Model file for the job. Use its own axes, mm. A direction names the side the tool comes from. Round coordinates to 2 decimals unless told otherwise and drop trailing zeros. Order: outer loops, then holes, each group sorted by start corner. A loop starts at its lowest first (then second) coordinate and runs counter-clockwise, first axis right, second up. Notation, with made-up numbers: (39.25, -25) - (50.25, -25) arc R33 ccw to (50.25, 6) - close; hole circle Ø9 at (-23.5, 86.5). An arc over 180 degrees is marked (long way). Answer as CSV lines item,"result". Start each with the question number.
1. 3-axis set-ups, long thin cutter, end or side, ignore diameter. For faces 4 (the face through (0, 3, -35)), 5 (the face through (49.78, 5.01, 37.05)), 6 (the face through (-38.28, 8.96, 89.19)): which of +Z, -Z, +X, -X, +Y, -Y reach the whole face in a straight line?
2. Band-saw the part on B-B on x = -22. List the corners of the cut face in (y, z), then the cut area to 3 significant figures.
3. Pin check, flat tips, straight feed: pin 1 Ø8 at (x, z) = (85.56, -41.72) entering from +Y; pin 2 Ø1.5 at (x, z) = (-43, -86.5) entering from +Y. Stop position of each tip, or through.
4. Wall check: line 1 along X through (y, z) = (4.6, 0); line 2 along X through (y, z) = (3.85, -75); line 3 along Y through (x, z) = (36.5, 39.5). Give the ranges that are in metal, low to high. Write a range as [from, to].
5. Band-saw the part on A-A on z = 11. List the corners of the cut face in (x, y), then the cut area to 3 significant figures.
6. Pull direction Z, two halves, no side cores. Call faces 1 (the face through (50.48, 8.96, 90.94)), 2 (the face through (-36.342, 8.958, 76.795)), 3 (the face through (-43, 12, -82)): released by +Z, released by -Z, zero draft, split by the parting line, or undercut.
```python
from build123d import *

# Parameters (mm, degrees)
SKETCH_1_W               = 200
SKETCH_1_H               = 200
SKETCH_1_R               = 2
EXTRUDE_1_DEPTH          = 6
CUT_EXTRUDE_1_DEPTH      = 2
FILLET_1_R               = 2
EXTRUDE_3_DEPTH          = 6
FILLET_4_R               = 40
SKETCH_4_R               = 2.5
CUT_EXTRUDE_2_DEPTH      = 8
SKETCH_7_R               = 9
SKETCH_7_W               = 18
SKETCH_7_H               = 8
SKETCH_7_W_2             = 8
SKETCH_7_H_2             = 18
CUT_EXTRUDE_3_DEPTH      = 6
CUT_EXTRUDE_4_DEPTH      = 2
FILLET_6_R               = 1
CUT_EXTRUDE_5_DEPTH      = 142.548578234
CUT_EXTRUDE_5_DEPTH_BACK = 142.548578234
SKETCH_9_R               = 35


with BuildPart() as part:
    # Эскиз1 → Бобышка-Вытянуть1 (new body)
    with BuildSketch(Plane(origin=(0, 0, 0), x_dir=(1, 0, 0), z_dir=(0, 1, 0))):
        Rectangle(SKETCH_1_W, SKETCH_1_H)
        with Locations(Location((-39.5, 75, 0), (0, 0, 270))):
            Circle(SKETCH_1_R, mode=Mode.SUBTRACT)
        with Locations(Location((39.5, 75, 0), (0, 0, 270))):
            Circle(SKETCH_1_R, mode=Mode.SUBTRACT)
        with Locations(Location((39.5, -75, 0), (0, 0, 270))):
            Circle(SKETCH_1_R, mode=Mode.SUBTRACT)
        with Locations(Location((-39.5, -75, 0), (0, 0, 270))):
            Circle(SKETCH_1_R, mode=Mode.SUBTRACT)
        with Locations(Location((39.5, 0, 0), (0, 0, 270))):
            Circle(SKETCH_1_R, mode=Mode.SUBTRACT)
        with Locations(Location((-39.5, 0, 0), (0, 0, 270))):
            Circle(SKETCH_1_R, mode=Mode.SUBTRACT)
        with Locations(Location((0, 39.5, 0), (0, 0, 270))):
            Circle(SKETCH_1_R, mode=Mode.SUBTRACT)
        with Locations(Location((0, -39.5, 0), (0, 0, 90))):
            Circle(SKETCH_1_R, mode=Mode.SUBTRACT)
        with Locations(Location((-75, 0, 0), (0, 0, 270))):
            Circle(SKETCH_1_R, mode=Mode.SUBTRACT)
        with Locations(Location((0, 75, 0), (0, 0, 270))):
            Circle(SKETCH_1_R, mode=Mode.SUBTRACT)
        with Locations(Location((75, 0, 0), (0, 0, 270))):
            Circle(SKETCH_1_R, mode=Mode.SUBTRACT)
        with Locations(Location((0, -75, 0), (0, 0, 270))):
            Circle(SKETCH_1_R, mode=Mode.SUBTRACT)
        with Locations(Location((-65, 65, 0), (0, 0, 270))):
            Circle(SKETCH_1_R, mode=Mode.SUBTRACT)
        with Locations(Location((65, 65, 0), (0, 0, 270))):
            Circle(SKETCH_1_R, mode=Mode.SUBTRACT)
        with Locations(Location((65, -65, 0), (0, 0, 270))):
            Circle(SKETCH_1_R, mode=Mode.SUBTRACT)
        with Locations(Location((-65, -65, 0), (0, 0, 270))):
            Circle(SKETCH_1_R, mode=Mode.SUBTRACT)
    extrude(amount=EXTRUDE_1_DEPTH)

    # Эскиз2 → Вырез-Вытянуть1 (cut)
    with BuildSketch(Plane(origin=(0, 6, 0), x_dir=(1, 0, 0), z_dir=(0, 1, 0))):
        Polygon((63.639610307, 33.941125497), (33.941125497, 63.639610307), (63.639610307, 93.338095117), (93.338095117, 63.639610307), align=None)
        Polygon((33.941125497, -63.639610307), (63.639610307, -33.941125497), (93.338095117, -63.639610307), (63.639610307, -93.338095117), align=None)
        Polygon((-63.639610307, -33.941125497), (-33.941125497, -63.639610307), (-63.639610307, -93.338095117), (-93.338095117, -63.639610307), align=None)
        Polygon((-33.941125497, 63.639610307), (-63.639610307, 33.941125497), (-93.338095117, 63.639610307), (-63.639610307, 93.338095117), align=None)
    extrude(amount=-CUT_EXTRUDE_1_DEPTH, mode=Mode.SUBTRACT)

    # Скругление1
    fillet_1_edges = [part.edges().sort_by_distance(p)[0] for p in [
        (-63.639610307, 5, 93.338095117),
        (-63.639610307, 5, -93.338095117),
        (-33.941125497, 5, -63.639610307),
        (-63.639610307, 5, -33.941125497),
        (-93.338095117, 5, -63.639610307),
        (63.639610307, 5, 93.338095117),
        (33.941125497, 5, 63.639610307),
        (63.639610307, 5, 33.941125497),
        (93.338095117, 5, 63.639610307),
        (93.338095117, 5, -63.639610307),
        (63.639610307, 5, -33.941125497),
        (33.941125497, 5, -63.639610307),
        (63.639610307, 5, -93.338095117),
        (-93.338095117, 5, 63.639610307),
        (-63.639610307, 5, 33.941125497),
        (-33.941125497, 5, 63.639610307),
    ]]
    fillet(fillet_1_edges, radius=FILLET_1_R)

    # Эскиз3 → Бобышка-Вытянуть3 (add)
    with BuildSketch(Plane(origin=(0, 6, 0), x_dir=(1, 0, 0), z_dir=(0, 1, 0))):
        Polygon((41.71930009, 71.4177849), (55.861435714, 85.559920524), (45.254833996, 96.166522241), (31.112698372, 82.024386618), align=None)
        Polygon((85.559920524, 55.861435714), (96.166522241, 45.254833996), (82.024386618, 31.112698372), (71.4177849, 41.71930009), align=None)
        Polygon((71.4177849, -41.71930009), (85.559920524, -55.861435714), (96.166522241, -45.254833996), (82.024386618, -31.112698372), align=None)
        Polygon((31.112698372, -82.024386618), (45.254833996, -96.166522241), (55.861435714, -85.559920524), (41.71930009, -71.4177849), align=None)
        Polygon((-41.71930009, -71.4177849), (-55.861435714, -85.559920524), (-45.254833996, -96.166522241), (-31.112698372, -82.024386618), align=None)
        Polygon((-85.559920524, -55.861435714), (-96.166522241, -45.254833996), (-82.024386618, -31.112698372), (-71.4177849, -41.71930009), align=None)
        Polygon((-71.4177849, 41.71930009), (-85.559920524, 55.861435714), (-96.166522241, 45.254833996), (-82.024386618, 31.112698372), align=None)
        Polygon((-31.112698372, 82.024386618), (-45.254833996, 96.166522241), (-55.861435714, 85.559920524), (-41.71930009, 71.4177849), align=None)
    extrude(amount=EXTRUDE_3_DEPTH)

    # Скругление4
    fillet_4_edges = [part.edges().sort_by_distance(p)[0] for p in [
        (100, 3, 100),
        (-100, 3, 100),
        (-100, 3, -100),
        (100, 3, -100),
    ]]
    fillet(fillet_4_edges, radius=FILLET_4_R)

    # Эскиз4 → Вырез-Вытянуть2 (cut)
    with BuildSketch(Plane(origin=(0, 12, 0), x_dir=(1, 0, 0), z_dir=(0, 1, 0))):
        with Locations(Location((41.71930009, 85.559920524, 0), (0, 0, 270))):
            Circle(SKETCH_4_R)
        with Locations(Location((85.559920524, 41.71930009, 0), (0, 0, 90))):
            Circle(SKETCH_4_R)
        with Locations(Location((85.559920524, -41.71930009, 0), (0, 0, 270))):
            Circle(SKETCH_4_R)
        with Locations(Location((41.71930009, -85.559920524, 0), (0, 0, 90))):
            Circle(SKETCH_4_R)
        with Locations(Location((-41.71930009, -85.559920524, 0), (0, 0, 270))):
            Circle(SKETCH_4_R)
        with Locations(Location((-85.559920524, -41.71930009, 0), (0, 0, 90))):
            Circle(SKETCH_4_R)
        with Locations(Location((-85.559920524, 41.71930009, 0), (0, 0, 270))):
            Circle(SKETCH_4_R)
        with Locations(Location((-41.71930009, 85.559920524, 0), (0, 0, 90))):
            Circle(SKETCH_4_R)
    extrude(amount=-CUT_EXTRUDE_2_DEPTH, mode=Mode.SUBTRACT)

    # Эскиз7 → Вырез-Вытянуть3 (cut)
    with BuildSketch(Plane(origin=(0, 6, 0), x_dir=(1, 0, 0), z_dir=(0, 1, 0))):
        with Locations(Location((21.213203436, 21.213203436, 0), (0, 0, 270))):
            Circle(SKETCH_7_R)
        with Locations(Location((21.213203436, -21.213203436, 0), (0, 0, 270))):
            Circle(SKETCH_7_R)
        with Locations(Location((-21.213203436, -21.213203436, 0), (0, 0, 270))):
            Circle(SKETCH_7_R)
        with Locations(Location((-21.213203436, 21.213203436, 0), (0, 0, 270))):
            Circle(SKETCH_7_R)
        with Locations((24, 0)):
            Rectangle(SKETCH_7_W, SKETCH_7_H)
        with Locations((0, 24)):
            Rectangle(SKETCH_7_W_2, SKETCH_7_H_2)
        with Locations((0, -24)):
            Rectangle(SKETCH_7_W_2, SKETCH_7_H_2)
        with Locations((-24, 0)):
            Rectangle(SKETCH_7_W, SKETCH_7_H)
    extrude(amount=-CUT_EXTRUDE_3_DEPTH, mode=Mode.SUBTRACT)

    # Эскиз8 → Вырез-Вытянуть4 (cut)
    with BuildSketch(Plane(origin=(0, 6, 0), x_dir=(1, 0, 0), z_dir=(0, 1, 0))):
        Polygon((44.547727215, 31.819805153), (31.819805153, 44.547727215), (53.033008589, 65.76093065), (65.76093065, 53.033008589), align=None)
        Polygon((65.76093065, -53.033008589), (53.033008589, -65.76093065), (31.819805153, -44.547727215), (44.547727215, -31.819805153), align=None)
        Polygon((-44.547727215, -31.819805153), (-31.819805153, -44.547727215), (-53.033008589, -65.76093065), (-65.76093065, -53.033008589), align=None)
        Polygon((-65.76093065, 53.033008589), (-53.033008589, 65.76093065), (-31.819805153, 44.547727215), (-44.547727215, 31.819805153), align=None)
    extrude(amount=-CUT_EXTRUDE_4_DEPTH, mode=Mode.SUBTRACT)

    # Скругление6
    fillet_6_edges = [part.edges().sort_by_distance(p)[0] for p in [
        (48.790367902, 12, -78.488852712),
        (78.488852712, 12, -48.790367902),
        (78.488852712, 12, 48.790367902),
        (48.790367902, 12, 78.488852712),
        (-48.790367902, 12, 78.488852712),
        (-78.488852712, 12, 48.790367902),
        (-78.488852712, 12, -48.790367902),
        (-48.790367902, 12, -78.488852712),
    ]]
    fillet(fillet_6_edges, radius=FILLET_6_R)

    # Эскиз9 → Вырез-Вытянуть5 (cut, two sides: drawn at the far end of the back side and taken through both)
    with BuildSketch(Plane(origin=(0, 6, 0), x_dir=(1, 0, 0), z_dir=(0, 1, 0)).offset(-CUT_EXTRUDE_5_DEPTH_BACK)):
        Circle(SKETCH_9_R)
    extrude(amount=CUT_EXTRUDE_5_DEPTH + CUT_EXTRUDE_5_DEPTH_BACK, mode=Mode.SUBTRACT)


solid = part.part
```
Reply:
1,face 4,"+Y, -Y"
1,face 5,"+Y"
1,face 6,"+Z, +Y"
2,outline,"(0, -100) - (6, -100) - (6, -30.18) - (0, -30.18) - close; (0, 30.18) - (6, 30.18) - (6, 100) - (0, 100) - close"
2,area,"838 mm2"
3,pin 1,"stops at y = 12"
3,pin 2,"stops at y = 4"
4,line 1,"x = [-100, -77], [-73, -41.5], [-37.5, -35], [35, 37.5], [41.5, 73], [77, 100]"
4,line 2,"x = [-97.08, -41.5], [-37.5, -2], [2, 37.5], [41.5, 97.08]"
4,line 3,"y = [0, 6]"
5,outline,"(-100, 0) - (-33.23, 0) - (-33.23, 6) - (-100, 6) - close; (33.23, 0) - (100, 0) - (100, 6) - (33.23, 6) - close"
5,area,"801 mm2"
6,face 1,"released by +Z"
6,face 2,"undercut"
6,face 3,"zero draft"
